from build123d import *

# Parameters (mm, degrees)
F0_R        = 3
F1_DEPTH    = 8
F2_R        = 10
F3_T1_DEPTH = 8
F4_R        = 1
F5_R        = 3.5
F6_DEPTH    = 55


# Not quite as in the source:
# - a fillet or chamfer that OpenCascade refuses, or shapes differently, is made with other operations: its cross-section is extruded or revolved along the edge and cut away or added


with BuildPart() as f1:
    # F0 (on Front) → F1 (new body)
    with BuildSketch(Plane.XZ):
        with BuildLine():
            Line((-7.5, 7), (-11.5, 7))
            Line((-11.5, 7), (-11.5, -7))
            Line((-11.5, -7), (-7.5, -7))
            ThreePointArc((-7.5, -7), (0, -10.2591422643), (7.5, -7))
            ThreePointArc((7.5, -7), (8.6053519278, -5.5855096632), (9.4472218138, -4))
            Line((9.4472218138, -4), (9.5, -4))
            Line((9.5, -4), (195, -4))
            Line((195, -4), (195, 4))
            Line((195, 4), (9.5, 4))
            Line((9.5, 4), (9.5, 7))
            Line((9.5, 7), (7.5, 7))
            ThreePointArc((7.5, 7), (7.2543090643, 7.2543090643), (7, 7.5))
            Line((7, 7.5), (7, 11.5))
            Line((7, 11.5), (-7, 11.5))
            Line((-7, 11.5), (-7, 7.5))
            ThreePointArc((-7, 7.5), (-7.2543090643, 7.2543090643), (-7.5, 7))
        make_face()
        Circle(F0_R, mode=Mode.SUBTRACT)
    extrude(amount=F1_DEPTH)

    # F2
    f2_edges = [f1.edges().sort_by_distance(p)[0] for p in [
        (9.447222, -4, -4),
    ]]
    fillet(f2_edges, radius=F2_R)

    # F3: fillet of radius 130 on 1 edges, made by hand

    # F3_s2 → F3_t1 (join)
    with BuildSketch(Plane.XZ):
        with BuildLine():
            ThreePointArc((37.2668867538, 4), (23.3026467101, 4.7521760338), (9.5, 7))
            Line((9.5, 7), (9.5, 4))
            Line((9.5, 4), (37.2668867538, 4))
        make_face()
    extrude(amount=F3_T1_DEPTH)

    # F4
    f4_edges = [f1.edges().sort_by_distance(p)[0] for p in [
        (7, -4, 11.5),
        (-7, -4, 11.5),
        (0, 0, 11.5),
        (0, -8, 11.5),
        (-11.5, -4, 7),
        (-11.5, -4, -7),
        (-11.5, 0, 0),
        (-11.5, -8, 0),
    ]]
    fillet(f4_edges, radius=F4_R)

    # F5 (on face) → F6 (join)
    with BuildSketch(Plane.YZ.offset(195)):
        with Locations((-4, 0)):
            Circle(F5_R)
    extrude(amount=F6_DEPTH)


solid = f1.part
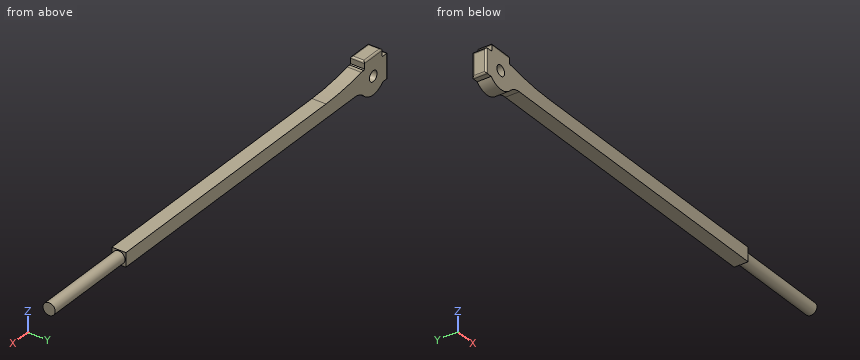
Check sheet for the modelled part. Datum: model origin and axes. Units: mm. Give positions to 0.01 mm unless a question says otherwise; leave off trailing zeros. Write each loop counter-clockwise with the first axis right and the second up, starting at its lowest first coordinate (ties: lowest second). Pieces come first, ordered by that corner, then holes. Notation, with made-up numbers: (1.5, 38.25) -> (56.5, 38.25) arc R24 ccw to (56.5, 74.25) -> close; hole circle Ø6 at (83.5, -1). An arc over 180 degrees is marked (long way). Use one line per item in the form item = value. Start each with the question number.
1. Thickness scan on line 1 along Z through (x, y) = (0, -2); line 2 along Z through (x, y) = (117.5, -6); line 3 along X through (y, z) = (-5.25, -1.25). Record the ranges inside material, lowest first. Write a range as from..to.
2. Section check B-B (z = 0). Record the cut outline in (x, y), and give its area (3 significant figures).
3. Section check A-A (x = 0). Record the cut outline in (y, z), and give its area (3 significant figures).
4. Section check C-C (x = 35). Record the cut outline in (y, z), and give its area (3 significant figures).
5. Go/stop test with flat-tipped pins: P1, Ø9.5, axis at x = 0, z = 0, coming from the -Y side; P2, Ø2.5, axis at y = -4, z = 9.5, coming from the -X side; P3, Ø2, axis at x = 171.5, y = -4, coming from the +Z side; P4, Ø1.6, axis at x = 8.5, y = -4.5, coming from the +Z side. Record where each tip stops, or that it passes through.
Conclusion:
q1.line_1 = -10.26..-3, 3..11.5
q1.line_2 = -4..4
q1.line_3 = -11.5..-2.73, 2.73..250
q2.outline = (-11.5, -7) arc R1 ccw to (-10.5, -8) -> (-3, -8) -> (-3, 0) -> (-10.5, 0) arc R1 ccw to (-11.5, -1) -> close; (3, -8) -> (195, -8) -> (195, -7.5) -> (250, -7.5) -> (250, -0.5) -> (195, -0.5) -> (195, 0) -> (3, 0) -> close
q2.area = 1,990 mm²
q3.outline = (-8, -10.26) -> (0, -10.26) -> (0, -3) -> (-8, -3) -> close; (-8, 3) -> (0, 3) -> (0, 10.5) arc R1 ccw to (-1, 11.5) -> (-7, 11.5) arc R1 ccw to (-8, 10.5) -> close
q3.area = 126 mm²
q4.outline = (-8, -4) -> (0, -4) -> (0, 4.02) -> (-8, 4.02) -> close
q4.area = 64.2 mm²
q5.P1 = -8
q5.P2 = -7
q5.P3 = 4
q5.P4 = 7
